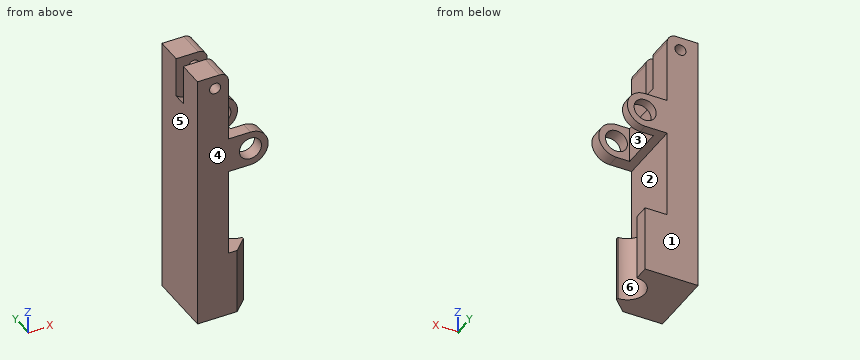
from build123d import *

# Parameters (mm, degrees)
SKETCH009_R       = 2.5
SKETCH009_R_2     = 1.25
PAD007_DEPTH      = 15
CYLINDER002_R     = 4
CYLINDER002_DEPTH = 27
CHAMFER001_SIZE2  = 3
CHAMFER001_SIZE   = 3
BOX_W             = 10
BOX_H             = 10.2
BOX_DEPTH         = 10
CYLINDER003_R     = 7
CYLINDER003_DEPTH = 3


with BuildPart() as part:
    # Sketch009 → Pad007 (new body)
    with BuildSketch(Plane.XZ):
        with BuildLine():
            Line((-12, 59.38), (-12, 0))
            Line((-12, 0), (0, 0))
            Line((0, 0), (0, 15))
            Line((0, 15), (-5, 15))
            Line((-5, 15), (-5, 35))
            Line((-5, 35), (0, 35))
            ThreePointArc((0, 35), (4, 39), (0, 43))
            Line((-5, 43), (0, 43))
            Line((-5, 43), (-5, 57.38))
            ThreePointArc((-5, 57.38), (-5.585786, 58.794214), (-7, 59.38))
            Line((-7, 59.38), (-12, 59.38))
        make_face()
        with Locations((0, 39)):
            Circle(SKETCH009_R, mode=Mode.SUBTRACT)
        with Locations((-8, 56.38)):
            Circle(SKETCH009_R_2, mode=Mode.SUBTRACT)
    extrude(amount=PAD007_DEPTH)

    # Cylinder002 → Cylinder002 (cut)
    with BuildSketch(Plane(origin=(0, -7.5, 0), x_dir=(1, 0, 0), z_dir=(0, 0, 1))):
        Circle(CYLINDER002_R)
    extrude(amount=CYLINDER002_DEPTH, mode=Mode.SUBTRACT)

    # Chamfer001
    chamfer001_edges = [part.edges().sort_by_distance(p)[0] for p in [
        (0, -15, 7.5),
    ]]
    chamfer001_side = part.faces().sort_by_distance((-7.04009, -15, 27.056502))[0]
    chamfer(chamfer001_edges, length=CHAMFER001_SIZE, length2=CHAMFER001_SIZE2, reference=chamfer001_side)

    # Box → Box (cut)
    with BuildSketch(Plane(origin=(-3, -12.1, 34), x_dir=(0, 1, 0), z_dir=(1, 0, 0))):
        with Locations((5, 5.1)):
            Rectangle(BOX_W, BOX_H)
    extrude(amount=BOX_DEPTH, mode=Mode.SUBTRACT)

    # Cylinder003 → Cylinder003 (cut)
    with BuildSketch(Plane(origin=(-8, -6, 56), x_dir=(1, 0, 0), z_dir=(0, -1, 0))):
        Circle(CYLINDER003_R)
    extrude(amount=CYLINDER003_DEPTH, mode=Mode.SUBTRACT)


solid = part.part
Geometry: final body of the model. Coordinates: model frame, mm. Face numbers are marked on the shaded views. A direction names the side the tool comes from. Give positions to 0.01 mm unless a question says otherwise; leave off trailing zeros. Loops run counter-clockwise (first coordinate to the right, second up) from the corner with the lowest first, then second, coordinate; pieces in that order, holes last. Notation, with made-up numbers: (69.25, 42.25) -> (118.25, 42.25) arc R10 ccw to (118.25, 58.25) -> close; hole circle Ø4 at (-26, 36). An arc over 180 degrees is marked (long way). Put each result on its own line as item: value.
1. Cut plane D-D (z = 14). Return the cut outline in (x, y).
Taken from the geometry:
outline: (-12, -15) -> (-3, -15) -> (0, -12) -> (0, -11.5) arc R4 cw to (0, -3.5) -> (0, 0) -> (-12, 0) -> close
2. Pull-direction query (Y, two-part tool) for the marked faces 4, 5 and 6; classes: released by +Y, released by -Y, zero draft, split by the parting line, or undercut.
Taken from the geometry:
face 4: released by -Y
face 5: zero draft
face 6: undercut
3. Cut plane A-A (z = 39). Return the cut outline in (x, y).
Taken from the geometry:
outline: (-12, -15) -> (-2.5, -15) -> (-2.5, -12.1) -> (-3, -12.1) -> (-3, -2.1) -> (-2.5, -2.1) -> (-2.5, 0) -> (-12, 0) -> close; (2.5, -15) -> (4, -15) -> (4, -12.1) -> (2.5, -12.1) -> close; (2.5, -2.1) -> (4, -2.1) -> (4, 0) -> (2.5, 0) -> close
4. Cut plane C-C (z = 56.38). Return the cut outline in (x, y).
Taken from the geometry:
outline: (-12, -15) -> (-9.25, -15) -> (-9.25, -9) -> (-12, -9) -> close; (-12, -6) -> (-9.25, -6) -> (-9.25, 0) -> (-12, 0) -> close; (-6.75, -15) -> (-5, -15) -> (-5, -9) -> (-6.75, -9) -> close; (-6.75, -6) -> (-5, -6) -> (-5, 0) -> (-6.75, 0) -> close
5. Cut plane B-B (x = -8). Return the cut outline in (y, z).
Taken from the geometry:
outline: (-15, 0) -> (0, 0) -> (0, 55.13) -> (-6, 55.13) -> (-6, 49) -> (-9, 49) -> (-9, 55.13) -> (-15, 55.13) -> close; (-15, 57.63) -> (-9, 57.63) -> (-9, 59.38) -> (-15, 59.38) -> close; (-6, 57.63) -> (0, 57.63) -> (0, 59.38) -> (-6, 59.38) -> close
6. Ray query, line 1 along X through (y, z) = (-4.4, 56.38); line 2 along Y through (x, z) = (-6, 56.5); line 3 along Z through (x, y) = (-4, -6.75). Return the intervals inside material, ascending. Write a range as [from, to].
Taken from the geometry:
line 1: x = [-12, -9.25], [-6.75, -5]
line 2: y = [-15, -9], [-6, 0]
line 3: z = [0, 15], [35, 43]
7. Set-up query: the marked faces 1, 2 and 3. Return all of +Z, -Z, +X, -X, +Y, -Y with unobstructed straight access to the full face (end or side cutting, diameter ignored); none if empty.
Taken from the geometry:
face 1: +Z, -Z, +X, -X, +Y
face 2: +X, +Y, -Y
face 3: +Z, +X
8. Pin query (flat end, axial travel): P1, Ø3, axis at x = 0, z = 39, coming from the +Y side; P2, Ø3, axis at x = -8, z = 56.38, coming from the +Y side; P3, Ø3, axis at y = -1.5, z = 4, coming from the +X side; P4, Ø2.5, axis at y = -8.5, z = 40.5, coming from the +X side. Return the tip coordinate at first contact, or that it passes through.
Taken from the geometry:
P1: passes through
P2: stops at y = 0
P3: stops at x = 0
P4: stops at x = -3
